```python
from build123d import *

# Parameters (mm, degrees)
SKETCH1_W               = 10
SKETCH1_H               = 13
SKETCH1_R               = 1.5
BOSS_EXTRUDE1_DEPTH     = 1
BOSS_EXTRUDE2_DEPTH     = 2
SKETCH3_RX              = 0.905906642
SKETCH3_RY              = 0.710654866
SKETCH3_R               = 0.45
BOSS_EXTRUDE3_DEPTH     = 1.25
SKETCH4_R               = 0.45
CUT_EXTRUDE1_DEPTH      = 3
CUT_EXTRUDE1_DEPTH_BACK = 2


with BuildPart() as part:
    # Sketch1 → Boss-Extrude1 (new body)
    with BuildSketch(Plane(origin=(0, 0, 0), x_dir=(1, 0, 0), z_dir=(0, 1, 0))):
        Rectangle(SKETCH1_W, SKETCH1_H)
        with Locations((-2.5, 4)):
            Circle(SKETCH1_R, mode=Mode.SUBTRACT)
    extrude(amount=BOSS_EXTRUDE1_DEPTH)

    # Sketch2 → Boss-Extrude2 (add)
    with BuildSketch(Plane(origin=(0, 0, 0), x_dir=(1, 0, 0), z_dir=(0, 1, 0))):
        with BuildLine():
            Line((1.25, 5.5), (2.75, 5.5))
            ThreePointArc((2.75, 5.5), (3.103553391, 5.353553391), (3.25, 5))
            Line((3.25, 5), (3.25, 3))
            ThreePointArc((3.25, 3), (3.103553391, 2.646446609), (2.75, 2.5))
            Line((2.75, 2.5), (1.25, 2.5))
            ThreePointArc((1.25, 2.5), (0.896446609, 2.646446609), (0.75, 3))
            Line((0.75, 3), (0.75, 5))
            ThreePointArc((0.75, 5), (0.896446609, 5.353553391), (1.25, 5.5))
        make_face()
    extrude(amount=BOSS_EXTRUDE2_DEPTH)

    # Sketch3 → Boss-Extrude3 (add)
    with BuildSketch(Plane(origin=(0, 0, 0), x_dir=(1, 0, 0), z_dir=(0, 1, 0))):
        with Locations(Location((-1.27, -5), (0, 0, -90))):
            Ellipse(SKETCH3_RX, SKETCH3_RY)
        with Locations((-1.27, -5)):
            Circle(SKETCH3_R, mode=Mode.SUBTRACT)
        with Locations(Location((-3.81, -5), (0, 0, -90))):
            Ellipse(SKETCH3_RX, SKETCH3_RY)
        with Locations((-3.81, -5)):
            Circle(SKETCH3_R, mode=Mode.SUBTRACT)
        with Locations(Location((3.81, -5), (0, 0, -90))):
            Ellipse(SKETCH3_RX, SKETCH3_RY)
        with Locations((3.81, -5)):
            Circle(SKETCH3_R, mode=Mode.SUBTRACT)
        with Locations(Location((1.27, -5), (0, 0, -90))):
            Ellipse(SKETCH3_RX, SKETCH3_RY)
        with Locations((1.27, -5)):
            Circle(SKETCH3_R, mode=Mode.SUBTRACT)
    extrude(amount=BOSS_EXTRUDE3_DEPTH)

    # Sketch4 → Cut-Extrude1 (cut, two sides)
    with BuildSketch(Plane(origin=(0, 0, 0), x_dir=(1, 0, 0), z_dir=(0, 1, 0))) as cut_extrude1_sk:
        with Locations((-3.81, -5)):
            Circle(SKETCH4_R)
        with Locations((-1.27, -5)):
            Circle(SKETCH4_R)
        with Locations((1.27, -5)):
            Circle(SKETCH4_R)
        with Locations((3.81, -5)):
            Circle(SKETCH4_R)
    extrude(amount=CUT_EXTRUDE1_DEPTH, mode=Mode.SUBTRACT)
    extrude(cut_extrude1_sk.sketch, amount=-CUT_EXTRUDE1_DEPTH_BACK, mode=Mode.SUBTRACT)


solid = part.part
```
Here's how the part is built. I have some questions about the finished solid (model axes, mm). A direction names the side the tool comes from. Coordinates: 2 decimals unless noted, no trailing zeros. Loops run counter-clockwise (first coordinate to the right, second up) from the corner with the lowest first, then second, coordinate; pieces in that order, holes last. Notation, with made-up numbers: (22.25, 1.5) -> (50.25, 1.5) arc R13 cw to (50.25, 18.5) -> close; hole circle Ø2 at (-15.5, 68). An arc over 180 degrees is marked (long way). Return JSON: item names as keys, results as strings.
1) If we section it at D-D, the plane y = 1.5: Write out the boundary of the cut face in (x, z).
Results below:
{"outline": "(0.75, -5) arc R0.5 ccw to (1.25, -5.5) -> (2.75, -5.5) arc R0.5 ccw to (3.25, -5) -> (3.25, -3) arc R0.5 ccw to (2.75, -2.5) -> (1.25, -2.5) arc R0.5 ccw to (0.75, -3) -> close"}
2) Thinking about a two-plate mould opening in X: for faces 1 (the face through (0, 0, 0)), 2 (the face through (1.211, 0.616, 4.554)), 3 (the face through (-5, 0.5, 0.1)), which applies, +X half, -X half, draft (parallel to the pull), parting line (faces both ways), or undercut?
Results below:
{"face 1": "draft", "face 2": "undercut", "face 3": "-X half"}
3) If we section it at B-B, the plane x = -2.5: Write out the boundary of the cut face in (y, z).
Results below:
{"outline": "(0, -6.5) -> (1, -6.5) -> (1, -5.5) -> (0, -5.5) -> close; (0, -2.5) -> (1, -2.5) -> (1, 6.5) -> (0, 6.5) -> close"}
4) Will these pins go through, and if not, where does the flat tip stop? pin 1 (1.6 mm diameter, centred on x = -3.5, z = 5, fed in from +Y); pin 2 (0.5 mm diameter, centred on y = 1.5, z = -3.5, fed in from +X); pin 3 (1 mm diameter, centred on x = -2, z = -2.5, fed in from +Y).
Results below:
{"pin 1": "y = 1.25", "pin 2": "x = 3.25", "pin 3": "y = 1"}
5) For faces 4 (the face through (2, 1.5, -5.5)), 5 (the face through (0.75, 1.5, -4)), 6 (the face through (3.25, 1.5, -4)), 7 (the face through (-3.6, 0.6, 4.6)), which set-ups out of +Z, -Z, +X, -X, +Y, -Y let a thin tool reach every point of the face, with its end or its side?
Results below:
{"face 4": "-Z, +X, -X, +Y", "face 5": "-Z, -X, +Y", "face 6": "-Z, +X, +Y", "face 7": "+Y, -Y"}
6) If we section it at C-C, the plane y = 0.55: Write out the boundary of the cut face in (x, z).
Results below:
{"outline": "(-5, -6.5) -> (5, -6.5) -> (5, 6.5) -> (-5, 6.5) -> close; hole circle Ø0.9 at (-3.81, 5); hole circle Ø3 at (-2.5, -4); hole circle Ø0.9 at (-1.27, 5); hole circle Ø0.9 at (1.27, 5); hole circle Ø0.9 at (3.81, 5)"}
7) If we section it at A-A, the plane z = -4: Write out the boundary of the cut face in (x, y).
Results below:
{"outline": "(-5, 0) -> (-4, 0) -> (-4, 1) -> (-5, 1) -> close; (-1, 0) -> (5, 0) -> (5, 1) -> (3.25, 1) -> (3.25, 2) -> (0.75, 2) -> (0.75, 1) -> (-1, 1) -> close"}
8) I need wall thicknesses on line 1 (X direction, y = 0.35, z = 5); line 2 (Z direction, x = -1.27, y = 0.7); line 3 (X direction, y = 0.5, z = -4). Which ranges of each line are inside material? Lowest first, please. Write a range as from..to.
Results below:
{"line 1": "-5..-4.26, -3.36..-1.72, -0.82..0.82, 1.72..3.36, 4.26..5", "line 2": "-6.5..-4.86, -3.14..4.55, 5.45..6.5", "line 3": "-5..-4, -1..5"}
